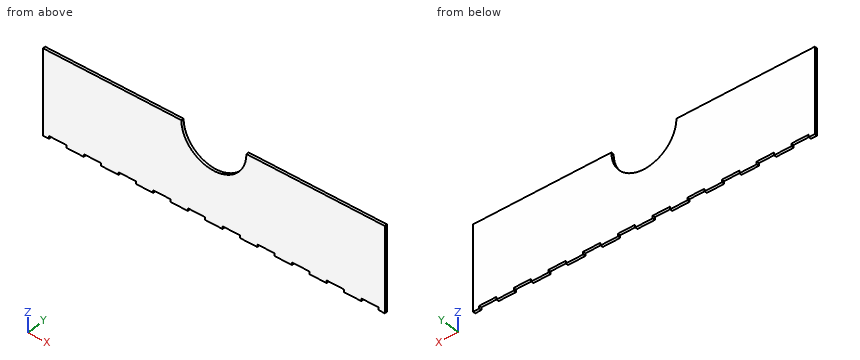
from build123d import *

# Parameters (mm, degrees)
F0_W     = 394
F0_H     = 94
F1_DEPTH = 3
F2_W     = 7
F2_H     = 3
F2_W_2   = 20
F3_DEPTH = 3
F4_R     = 37.5
F5_DEPTH = 25


with BuildPart() as f1:
    # F0 (on Front) → F1 (new body)
    with BuildSketch(Plane.XZ):
        Rectangle(F0_W, F0_H)
    extrude(amount=F1_DEPTH)

    # F2 (on face) → F3 (join, through all)
    with BuildSketch(Plane.XZ.offset(3)):
        with Locations((-193.5, -48.5)):
            Rectangle(F2_W, F2_H)
        with Locations((193.5, -48.5)):
            Rectangle(F2_W, F2_H)
        with Locations((-160, -48.5)):
            Rectangle(F2_W_2, F2_H)
        with Locations((-120, -48.5)):
            Rectangle(F2_W_2, F2_H)
        with Locations((-80, -48.5)):
            Rectangle(F2_W_2, F2_H)
        with Locations((-40, -48.5)):
            Rectangle(F2_W_2, F2_H)
        with Locations((0, -48.5)):
            Rectangle(F2_W_2, F2_H)
        with Locations((40, -48.5)):
            Rectangle(F2_W_2, F2_H)
        with Locations((80, -48.5)):
            Rectangle(F2_W_2, F2_H)
        with Locations((120, -48.5)):
            Rectangle(F2_W_2, F2_H)
        with Locations((160, -48.5)):
            Rectangle(F2_W_2, F2_H)
    extrude(amount=-F3_DEPTH)

    # F4 (on face) → F5 (cut)
    with BuildSketch(Plane.XZ.offset(3)):
        with Locations((0, 47)):
            Circle(F4_R)
    extrude(amount=-F5_DEPTH, mode=Mode.SUBTRACT)


solid = f1.part
Here's how the part is built. I have some questions about the finished solid (model axes, mm). Give positions to 0.01 mm unless a question says otherwise; leave off trailing zeros. Write each loop counter-clockwise with the first axis right and the second up, starting at its lowest first coordinate (ties: lowest second). Pieces come first, ordered by that corner, then holes. Notation, with made-up numbers: (1.5, 40.25) -> (56.5, 40.25) arc R35 ccw to (56.5, 73.25) -> close; hole circle Ø3 at (37.5, -25.75). An arc over 180 degrees is marked (long way). Use one line per item in the form item = value. Start each with the question number.
1. Imagine slicing it at A-A on x = 0. List the corners of the cut face in (y, z) for me, plus the area to 4 significant figures.
2. Imagine slicing it at B-B on x = 135. List the corners of the cut face in (y, z) for me, plus the area to 3 significant figures.
3. If I drill on L1, parallel to Z at x = 51, y = -0.95; L2, parallel to X at y = -1.3, z = 15.5; L3, parallel to X at y = -2.5, z = 26, over which ranges is the centre line in solid material (lowest first)?
4. Will this pin go through, and if not, where does the flat tip stop? pin 1 Ø0.9 at (x, y) = (16.5, -2) entering from -Z.
Entries:
q1.outline = (-3, -50) -> (0, -50) -> (0, 9.5) -> (-3, 9.5) -> close
q1.area = 178.5 mm²
q2.outline = (-3, -47) -> (0, -47) -> (0, 47) -> (-3, 47) -> close
q2.area = 282 mm²
q3.L1 = -47 to 47
q3.L2 = -197 to -20.35, 20.35 to 197
q3.L3 = -197 to -31.07, 31.07 to 197
q4.pin_1 = -47
